Autodesk Inventor part; units mm, degrees
ref_plane "YZ Plane" through (0, 0, 0) normal (1, 0, 0) x (0, 1, 0)
ref_plane "XZ Plane" through (0, 0, 0) normal (0, 1, 0) x (-1, 0, 0)
ref_plane "XY Plane" through (0, 0, 0) normal (0, 0, 1) x (1, 0, 0)
sketch "Sketch1" plane through (0, 0, 0) normal (0, 1, 0) x (-1, 0, 0)
  line L0 (4.8, 4.8) -> (-4.8, 4.8)
  line L1 (-4.8, 4.8) -> (-4.8, -4.8)
  line L2 (-4.8, -4.8) -> (4.8, -4.8)
  line L3 (4.8, -4.8) -> (4.8, 4.8)
  point P0 (0, 0)
  point P1 (4.8, 0)
  point P2 (0, -4.8)
  dimension "d0" = 9.6
  dimension "d1" = 9.6
extrude "Extrusion1" add sketch "Sketch1" along normal blind 35
sketch "Sketch5" plane through (0, 0, 0) normal (0, -1, 0) x (1, 0, 0)
  circle A0 centre (0, 0) radius 1.75
  line L0 (4.8, 4.8) -> (4.8, -4.8)
  line L1 (-4.8, 4.8) -> (4.8, 4.8)
  line L2 (4.8, -4.8) -> (-4.8, -4.8)
  line L3 (4.8, 4.8) -> (-4.8, 4.8)
  line L4 (-4.8, 4.8) -> (-4.8, -4.8)
  line L5 (-4.8, -4.8) -> (4.8, -4.8)
  line L6 (4.8, -4.8) -> (4.8, 4.8)
  circle A1 centre (0, 0) radius 6.7882
  point P0 (-4.8, 4.8)
  point P1 (-4.8, 4.8)
  point P2 (-4.8, 4.8)
  dimension "d14" = 3.5
extrude "Extrusion5" add sketch "Sketch5" against normal blind 10 contours A1 L0 | L1 A1 | A1 L2 | L4 A1
sketch "Sketch6" plane through (4.8, 35, 4.8) normal (1, 0, 0) x (0, 0, -1)
  line L0 (0, 0) -> (9.6, 0)
  point P0 (4.8, -35)
  point P1 (4.8, -3.5)
  point P2 (4.8, 0)
  dimension "d18" = 3.5
hole "Hole1" at (4.8, 31.5, 0) direction (-1, 0, 0) diameter 1.5 end through all
sketch "Sketch9" plane through (4.8, 35, 4.8) normal (1, 0, 0) x (0, 0, -1)
  circle A0 centre (4.8, -30) radius 1.75
  point P0 (4.8, -35)
  dimension "d41" = 5
  dimension "d42" = 3.5
extrude "Extrusion7" cut sketch "Sketch9" along normal blind 5 and the other way blind 4
sketch "Sketch10" plane through (0, 0, 0) normal (0, -1, 0) x (1, 0, 0)
  point P0 (0, 0)
  point P1 (0, 0)
hole "Hole3" at (0, 0, 0) direction (0, 1, 0) diameter 3.5 depth 9 tip angle 118
sketch "Sketch11" plane through (0, 0, 0) normal (0, -1, 0) x (1, 0, 0)
  circle A0 centre (0, 0) radius 5
  circle A1 centre (0, 0) radius 7.5
  dimension "d55" = 10
  dimension "d63" = 15
extrude "Extrusion8" cut sketch "Sketch11" against normal blind 2
fillet "Fillet3" radius 2 1 edges at (-5, 2, 0)
chamfer "Chamfer1" distance 2 angle 45 4 edges at (-4.8, 35, 0) (0, 35, -4.8) (4.8, 35, 0) (0, 35, 4.8)
fillet "Fillet5" radius 1 2 edges at (6.2715, 2, -2.5977) (-6.2715, 2, 2.5977)
properties part number "wheel-lockV2"
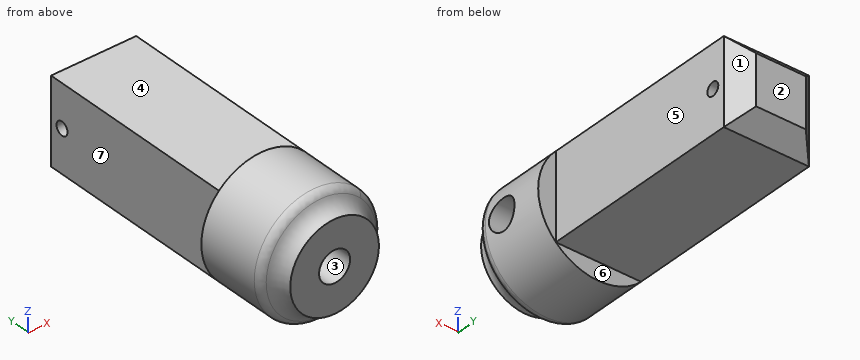
Geometry: final body of the model. Coordinates: model frame, mm. Face numbers are marked on the shaded views. A direction names the side the tool comes from. Give positions to 0.01 mm unless a question says otherwise; leave off trailing zeros. Write each loop counter-clockwise with the first axis right and the second up, starting at its lowest first coordinate (ties: lowest second). Pieces come first, ordered by that corner, then holes. Notation, with made-up numbers: M 1.25,-27 L 32.25,-27 A17 cw 32.25,0 Z; hole C 10,20 d8. An arc over 180 degrees is marked long. Answer in a Markdown table with one row per item. Add a question column.
(1) Section B-B on y = 14. Return loops of the section in (x, z), and give its area (3 significant figures).
(2) Section C-C on y = 5. Return loops of the section in (x, z), and give its area (3 significant figures).
(3) Ray query, line 1 (Z direction, x = 0.75, y = 13); line 2 (Z direction, x = 2, y = 31.5). Return the intervals inside material, ascending.
(4) Section A-A on y = 31.5. Return loops of the section in (x, z), and give its area (3 significant figures).
(5) Mould query, pull axis X, two halves, no side actions, for the marked faces 1, 2 and 3. Classes: +X half, -X half, draft (parallel to the pull), parting line (faces both ways), or undercut.
(6) Reachability of the marked faces 4, 5, 6 and 7 from +Z, -Z, +X, -X, +Y, -Y: full face, straight path, thin tool, end or side. Return the list, or none.
(7) First-contact query: pin 1 (8 mm diameter, centred on y = 17, z = -4.5, fed in from -X); pin 2 (1 mm diameter, centred on x = 2.5, z = 6, fed in from +Y); pin 3 (5 mm diameter, centred on x = 0.5, y = 17, fed in from +Z). Flat tips, straight axial feed; report the tip coordinate or a pass-through.
Result set:
| question | item | result |
|---|---|---|
| 1 | outline | M -4.8,-4.8 L 4.8,-4.8 L 4.8,4.8 L -4.8,4.8 Z |
| 1 | area | 92.2 mm^2 |
| 2 | outline | M 0.8,-1.75 L 0.8,-1.56 A1.75 cw long 0.8,1.56 L 0.8,1.75 L 6.56,1.75 A6.79 ccw long 6.56,-1.75 Z |
| 2 | area | 117 mm^2 |
| 3 | line 1 | z = -4.8 to 4.8 |
| 3 | line 2 | z = -4.8 to -0.75, 0.75 to 4.8 |
| 4 | outline | M -4.8,-4.8 L 4.8,-4.8 L 4.8,-0.75 L -4.8,-0.75 Z; M -4.8,0.75 L 4.8,0.75 L 4.8,4.8 L -4.8,4.8 Z |
| 4 | area | 77.8 mm^2 |
| 5 | face 1 | +X half |
| 5 | face 2 | draft |
| 5 | face 3 | undercut |
| 6 | face 4 | +Z, +X, -X, +Y |
| 6 | face 5 | +Z, -Z, +X, +Y |
| 6 | face 6 | -Z, +X, -X, +Y |
| 6 | face 7 | +Z, -Z, -X, +Y |
| 7 | pin 1 | stops at x = -4.8 |
| 7 | pin 2 | stops at y = 10 |
| 7 | pin 3 | stops at z = 4.8 |
